Autodesk Inventor part; units mm, degrees
ref_plane "YZ Plane" through (0, 0, 0) normal (1, 0, 0) x (0, 1, 0)
ref_plane "XZ Plane" through (0, 0, 0) normal (0, 1, 0) x (-1, 0, 0)
ref_plane "XY Plane" through (0, 0, 0) normal (0, 0, 1) x (1, 0, 0)
sketch "Sketch1" plane through (0, 0, 0) normal (1, 0, 0) x (0, 1, 0)
  line L0 (-20, -30) -> (20, -30)
  line L1 (20, -30) -> (20, 30)
  line L2 (20, 30) -> (-20, 30)
  line L3 (-20, 30) -> (-20, -30)
  line L4 (-20, -30) -> (20, 30) construction
  line L5 (20, -30) -> (-20, 30) construction
  circle A0 centre (0, -30) radius 20
  point P0 (0, 0)
  dimension "d0" = 40
  dimension "d1" = 60
extrude "Extrusion1" add sketch "Sketch1" along normal blind 3.6
sketch "Sketch4" plane through (3.6, 0, 0) normal (1, 0, 0) x (0, 0, -1)
  line L0 (-5, 20) -> (-55, 20)
  line L1 (-55, 20) -> (-55, -20)
  line L2 (-55, -20) -> (-5, -20)
  line L3 (-5, -20) -> (-5, 20)
  line L4 (0, -64) -> (0, 34)
  line L5 (-10, -75.9609) -> (-10, 61.6)
  line L6 (30, 20) -> (-30, 20)
  dimension "d40" = 50
  dimension "d41" = 40
  dimension "d50" = 10
  dimension "d51" = 5
  dimension "d53" = 0
extrude "Extrusion4" add sketch "Sketch4" against normal blind 3.6
sketch "Sketch5" plane through (0, 0, 0) normal (-1, 0, 0) x (0, 0, 1)
  line L0 (52, -47) -> (41.7, -47)
  line L1 (41.7, -47) -> (41.7, -42.7)
  line L2 (41.7, -42.7) -> (52, -42.7)
  line L3 (52, -42.7) -> (52, -47)
  line L4 (55, -20) -> (55, -6.689)
  line L5 (55, -20) -> (55, 20)
  line L6 (55, -50) -> (10.2215, -50)
  line L7 (5, -50) -> (55, -50)
  point P0 (10.2215, -50)
  dimension "d20" = 10.3
  dimension "d21" = 4.3
  dimension "d42" = 3
  dimension "d43" = 3
extrude "Extrusion5" cut sketch "Sketch5" against normal blind 4
sketch "Sketch2" plane through (0, 0, 0) normal (-1, 0, 0) x (0, 0, 1)
  arc A0 (-30, 20) -> (-30, -20) centre (-30, 0) ccw
  circle A1 centre (-30, 0) radius 5.15
  point P0 (0, 0)
  dimension "d4" = 10.3
extrude "Extrusion2" cut sketch "Sketch2" against normal blind 4
fillet "Fillet3" [suppressed]
properties part number "houder"
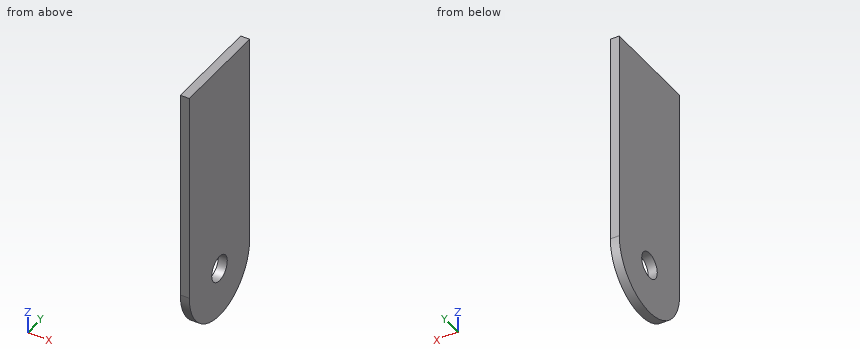
Here's how the part is built. I have some questions about the finished solid (model axes, mm). Give positions to 0.01 mm unless a question says otherwise; leave off trailing zeros. Loops run counter-clockwise (first coordinate to the right, second up) from the corner with the lowest first, then second, coordinate; pieces in that order, holes last. Notation, with made-up numbers: (45, 60.5) -> (94, 60.5) arc R14 ccw to (94, 74.5) -> close; hole circle Ø1 at (-3, 52). An arc over 180 degrees is marked (long way). Answer as a JSON object with one key per item and string values. Group by question number.
Item 1: Imagine slicing it at B-B on x = 0.8. Write out the boundary of the cut face in (y, z).
Item 2: Imagine slicing it at A-A on y = 0. Write out the boundary of the cut face in (x, z).
Item 3: I need wall thicknesses on L1, parallel to Y at x = 1.7, z = -30; L2, parallel to Z at x = 1.2, y = -3; L3, parallel to Z at x = 1.05, y = 4. Which ranges of each line are inside material? Lowest first, please.
Item 4: Imagine slicing it at D-D on y = -16. Write out the boundary of the cut face in (x, z).
Item 5: Imagine slicing it at C-C on z = -34. Write out the boundary of the cut face in (x, y).
Answer list:
{
 "1": {"outline": "(-20, -30) arc R20 ccw to (20, -30) -> (20, 55) -> (-20, 55) -> close; hole circle Ø10.3 at (0, -30)"},
 "2": {"outline": "(0, -50) -> (3.6, -50) -> (3.6, -35.15) -> (0, -35.15) -> close; (0, -24.85) -> (3.6, -24.85) -> (3.6, 55) -> (0, 55) -> close"},
 "3": {"L1": "y = -20 to -5.15, 5.15 to 20", "L2": "z = -49.77 to -34.19, -25.81 to 55", "L3": "z = -49.6 to -33.24, -26.76 to 55"},
 "4": {"outline": "(0, -42) -> (3.6, -42) -> (3.6, 55) -> (0, 55) -> close"},
 "5": {"outline": "(0, -19.6) -> (3.6, -19.6) -> (3.6, -3.24) -> (0, -3.24) -> close; (0, 3.24) -> (3.6, 3.24) -> (3.6, 19.6) -> (0, 19.6) -> close"}
}
